from build123d import *

# Parameters (mm, degrees)
SKETCH1_W           = 62.3
SKETCH1_H           = 42.3
BOSS_EXTRUDE1_DEPTH = 5
SKETCH2_W           = 5
SKETCH2_H           = 42.3
BOSS_EXTRUDE2_DEPTH = 42.3
SKETCH3_W           = 47.3
SKETCH3_H           = 42.3
SKETCH3_R           = 11
BOSS_EXTRUDE3_DEPTH = 5
SKETCH4_R           = 1.5
CUT_EXTRUDE1_DEPTH  = 5
SKETCH5_R           = 1.5
CUT_EXTRUDE2_DEPTH  = 5
SKETCH6_W           = 66.403823896
SKETCH6_H           = 55.517872021
CUT_EXTRUDE3_DEPTH  = 40


with BuildPart() as part:
    # Sketch1 → Boss-Extrude1 (new body)
    with BuildSketch(Plane(origin=(0, 0, 0), x_dir=(1, 0, 0), z_dir=(0, 1, 0))):
        with Locations((31.15, 21.15)):
            Rectangle(SKETCH1_W, SKETCH1_H)
    extrude(amount=BOSS_EXTRUDE1_DEPTH)

    # Sketch2 → Boss-Extrude2 (add)
    with BuildSketch(Plane(origin=(0, 5, 0), x_dir=(1, 0, 0), z_dir=(0, 1, 0))):
        with Locations((2.5, 21.15)):
            Rectangle(SKETCH2_W, SKETCH2_H)
    extrude(amount=BOSS_EXTRUDE2_DEPTH)

    # Sketch3 → Boss-Extrude3 (add)
    with BuildSketch(Plane(origin=(0, 47.3, 0), x_dir=(1, 0, 0), z_dir=(0, 1, 0))):
        with Locations((23.65, 21.15)):
            Rectangle(SKETCH3_W, SKETCH3_H)
        with Locations(Location((26.15, 21.15, 0), (0, 0, 270))):
            Circle(SKETCH3_R, mode=Mode.SUBTRACT)
    extrude(amount=BOSS_EXTRUDE3_DEPTH)

    # Sketch4 → Cut-Extrude1 (cut)
    with BuildSketch(Plane(origin=(0, 52.3, 0), x_dir=(1, 0, 0), z_dir=(0, 1, 0))):
        with Locations(Location((41.65, 36.65, 0), (0, 0, 270))):
            Circle(SKETCH4_R)
        with Locations(Location((10.65, 36.65, 0), (0, 0, 270))):
            Circle(SKETCH4_R)
        with Locations(Location((10.65, 5.65, 0), (0, 0, 270))):
            Circle(SKETCH4_R)
        with Locations(Location((41.65, 5.65, 0), (0, 0, 270))):
            Circle(SKETCH4_R)
    extrude(amount=-CUT_EXTRUDE1_DEPTH, mode=Mode.SUBTRACT)

    # Sketch5 → Cut-Extrude2 (cut)
    with BuildSketch(Plane(origin=(0, 5, 0), x_dir=(1, 0, 0), z_dir=(0, 1, 0))):
        with Locations(Location((55.3, 5.5, 0), (0, 0, 270))):
            Circle(SKETCH5_R)
        with Locations(Location((55.3, 36.8, 0), (0, 0, 270))):
            Circle(SKETCH5_R)
    extrude(amount=-CUT_EXTRUDE2_DEPTH, mode=Mode.SUBTRACT)

    # Sketch6 → Cut-Extrude3 (cut)
    with BuildSketch(Plane(origin=(0, 0, -21.15), x_dir=(-1, 0, 0), z_dir=(0, 0, -1))):
        with Locations((-30.988329777, 26.343035963)):
            Rectangle(SKETCH6_W, SKETCH6_H)
    extrude(amount=-CUT_EXTRUDE3_DEPTH, mode=Mode.SUBTRACT)


solid = part.part
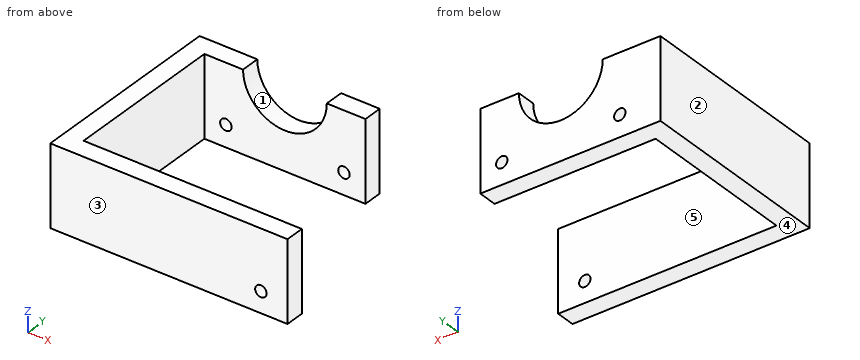
The model under review builds one solid part; all positions refer to its coordinate system, in mm. Face numbers are marked on the shaded views. A direction names the side the tool comes from. Give positions to 0.01 mm unless a question says otherwise; leave off trailing zeros. Loops run counter-clockwise (first coordinate to the right, second up) from the corner with the lowest first, then second, coordinate; pieces in that order, holes last. Notation, with made-up numbers: (-39, 58.25) -> (-17, 58.25) arc R8 cw to (-17, 64.25) -> close; hole circle Ø6 at (40.25, 77.25). An arc over 180 degrees is marked (long way). Put each result on its own line as item: value. Start each with the question number.
1. Wall thickness on probe 1 along X at (y, z) = (49.85, -36.65); probe 2 along Y at (x, z) = (13, -24.75); probe 3 along Y at (x, z) = (52.5, -35.5): over which ranges is each line inside the solid? List them lowest first.
2. We need section C-C on x = 41.65. State the section outline as (y, z) points.
3. We need section A-A on x = 26.15. State the section outline as (y, z) points, then the cut area to 4 significant figures.
4. Mouldability with a two-part tool opening along X and no side actions: class the marked faces 1, 2 and 3 as released by +X, released by -X, zero draft, split by the parting line, or undercut.
5. We need section D-D on z = -36.8. State the section outline as (x, y) points, then the cut area to 3 significant figures.
6. Clearance check with flat-ended pins moving along their axes: P1, Ø2, axis at y = 38, z = -36.5, coming from the +X side; P2, Ø4, axis at x = 55.3, z = -36.8, coming from the +Y side; P3, Ø12, axis at x = 19, y = 16.5, coming from the +Z side; P4, Ø2.5, axis at y = 50.5, z = -33, coming from the +X side. State where each tip first meets the part, or that it passes through.
7. For the marked faces 4 and 5, list the 3-axis set-ups (+Z, -Z, +X, -X, +Y, -Y) from which the entire face can be reached by the end or side of a thin tool; tool diameter is ignored.
8. We need section B-B on z = -27. State the section outline as (x, y) points, then the cut area to 3 significant figures.
Determined:
1. probe 1: 0 to 9.15, 12.15 to 40.15, 43.15 to 47.3
1. probe 2: 0 to 5, 47.3 to 52.3
1. probe 3: 0 to 5
2. outline: (0, -42.3) -> (5, -42.3) -> (5, -21.15) -> (0, -21.15) -> close; (47.3, -42.3) -> (52.3, -42.3) -> (52.3, -38.15) -> (47.3, -38.15) -> close; (47.3, -35.15) -> (52.3, -35.15) -> (52.3, -21.15) -> (47.3, -21.15) -> close
3. outline: (0, -42.3) -> (5, -42.3) -> (5, -21.15) -> (0, -21.15) -> close; (47.3, -42.3) -> (52.3, -42.3) -> (52.3, -32.15) -> (47.3, -32.15) -> close
3. area: 156.5 mm^2
4. face 1: undercut
4. face 2: released by -X
4. face 3: zero draft
5. outline: (0, 0) -> (53.8, 0) -> (53.8, 5) -> (5, 5) -> (5, 47.3) -> (9.16, 47.3) -> (9.16, 52.3) -> (0, 52.3) -> close; (12.14, 47.3) -> (40.16, 47.3) -> (40.16, 52.3) -> (12.14, 52.3) -> close; (43.14, 47.3) -> (47.3, 47.3) -> (47.3, 52.3) -> (43.14, 52.3) -> close; (56.8, 0) -> (62.3, 0) -> (62.3, 5) -> (56.8, 5) -> close
5. area: 715 mm^2
6. P1: x = 5
6. P2: y = 5
6. P3: through
6. P4: x = 47.3
7. face 4: -Z, +X, -X, +Y, -Y
7. face 5: +Z, -Z, +X
8. outline: (0, 0) -> (62.3, 0) -> (62.3, 5) -> (5, 5) -> (5, 47.3) -> (16.83, 47.3) -> (16.83, 52.3) -> (0, 52.3) -> close; (35.47, 47.3) -> (47.3, 47.3) -> (47.3, 52.3) -> (35.47, 52.3) -> close
8. area: 666 mm^2
